Source: CAD feature listing. Evaluate the final solid. Frame: model axes, mm. Give positions to 0.01 mm unless a question says otherwise; leave off trailing zeros. Write each loop counter-clockwise with the first axis right and the second up, starting at its lowest first coordinate (ties: lowest second). Pieces come first, ordered by that corner, then holes. Notation, with made-up numbers: (-14.75, 3.5) -> (38.25, 3.5) arc R11 ccw to (38.25, 9.5) -> close; hole circle Ø8 at (41.5, -17.75). An arc over 180 degrees is marked (long way). Use a Markdown table: item, result. Add a question column.
Autodesk Inventor part; units mm, degrees
ref_plane "YZ Plane" through (0, 0, 0) normal (1, 0, 0) x (0, 1, 0)
ref_plane "XZ Plane" through (0, 0, 0) normal (0, 1, 0) x (-1, 0, 0)
ref_plane "XY Plane" through (0, 0, 0) normal (0, 0, 1) x (1, 0, 0)
sketch "Sketch1" plane through (0, 0, 0) normal (0, 1, 0) x (-1, 0, 0)
  line L0 (-10.0391, 0) -> (-100.3906, 0)
  line L1 (-110.4297, -10.0391) -> (-110.4297, -100.3906)
  line L2 (-100.3906, -110.4297) -> (-10.0391, -110.4297)
  line L3 (0, -100.3906) -> (0, -10.0391)
  arc A0 (-10.0391, -110.4297) -> (0, -100.3906) centre (-10.0391, -100.3906) ccw
  arc A1 (-110.4297, -100.3906) -> (-100.3906, -110.4297) centre (-100.3906, -100.3906) ccw
  arc A2 (-100.3906, 0) -> (-110.4297, -10.0391) centre (-100.3906, -10.0391) ccw
  arc A3 (0, -10.0391) -> (-10.0391, 0) centre (-10.0391, -10.0391) ccw
  line L4 (-23.0414, -4.0156) -> (-87.3883, -4.0156)
  line L5 (-106.4141, -23.0414) -> (-106.4141, -87.3883)
  line L6 (-87.3883, -106.4141) -> (-23.0414, -106.4141)
  line L7 (-4.0156, -87.3883) -> (-4.0156, -23.0414)
  circle A4 centre (-7.3285, -7.3285) radius 2.0078
  circle A5 centre (-7.3285, -103.1012) radius 2.0078
  circle A6 centre (-103.1012, -103.1012) radius 2.0078
  circle A7 centre (-103.1012, -7.3285) radius 2.0078
  line L8 (-6.3588, -17.3846) -> (-17.3846, -6.3588)
  line L9 (-93.0451, -6.3588) -> (-104.0709, -17.3846)
  line L10 (-104.0709, -93.0451) -> (-93.0451, -104.0709)
  line L11 (-17.3846, -104.0709) -> (-6.3588, -93.0451)
  arc A8 (-17.3846, -6.3588) -> (-23.0414, -4.0156) centre (-23.0414, -12.0156) ccw
  arc A9 (-4.0156, -23.0414) -> (-6.3588, -17.3846) centre (-12.0156, -23.0414) ccw
  arc A10 (-6.3588, -93.0451) -> (-4.0156, -87.3883) centre (-12.0156, -87.3883) ccw
  arc A11 (-23.0414, -106.4141) -> (-17.3846, -104.0709) centre (-23.0414, -98.4141) ccw
  arc A12 (-93.0451, -104.0709) -> (-87.3883, -106.4141) centre (-87.3883, -98.4141) ccw
  arc A13 (-106.4141, -87.3883) -> (-104.0709, -93.0451) centre (-98.4141, -87.3883) ccw
  arc A14 (-104.0709, -17.3846) -> (-106.4141, -23.0414) centre (-98.4141, -23.0414) ccw
  arc A15 (-87.3883, -4.0156) -> (-93.0451, -6.3588) centre (-87.3883, -12.0156) ccw
  point P0 (0, 0)
  point P1 (-4.0156, -4.0156)
  point P2 (-106.4141, -106.4141)
  point P3 (-106.4141, -4.0156)
  point P4 (-4.0156, -106.4141)
  point P5 (-4.0156, -19.7277)
  point P6 (-19.7277, -4.0156)
  point P7 (-55.2148, -55.2148)
  point P8 (-90.702, -4.0156)
  point P9 (-106.4141, -19.7277)
  point P10 (-106.4141, -90.702)
  point P11 (-90.702, -106.4141)
  point P12 (-19.7277, -106.4141)
  point P13 (-4.0156, -90.702)
  dimension "d25" = 360
extrude "Extrusion1" add sketch "Sketch1" along normal blind 3.2
properties part number "Spacer"
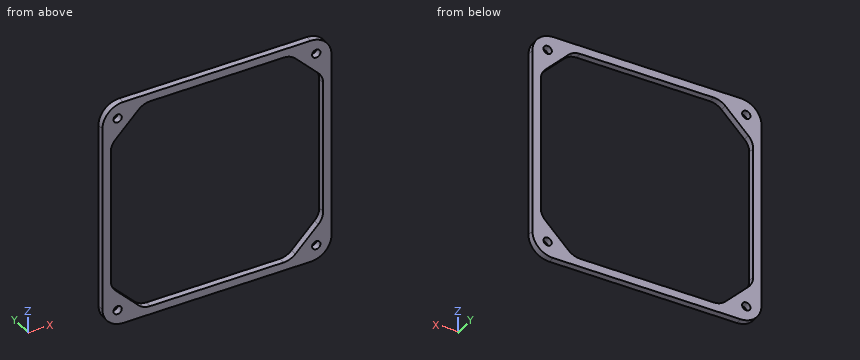
(1) Cut plane A-A on x = 66. Return the cut outline in (y, z).
(2) Material intervals for L1, parallel to X at y = 1.8, z = -79.5; L2, parallel to Z at x = 50, y = 2.75; L3, parallel to X at y = 0.2, z = -102.5, sorted ascending.
(3) Cut plane B-B on z = -28. Return the cut outline in (x, y), then the cut area to 3 significant figures.
(4) Cut plane C-C on y = 1.3. Return the cut outline in (x, z), then the cut area to 3 significant figures.
Output:
| question | item | result |
|---|---|---|
| 1 | outline | (0, -110.43) -> (3.2, -110.43) -> (3.2, -106.41) -> (0, -106.41) -> close; (0, -4.02) -> (3.2, -4.02) -> (3.2, 0) -> (0, 0) -> close |
| 2 | L1 | 0 to 4.02, 106.41 to 110.43 |
| 2 | L2 | -110.43 to -106.41, -4.02 to 0 |
| 2 | L3 | 0.22 to 5.41, 9.24 to 15.81, 94.62 to 101.19, 105.02 to 110.21 |
| 3 | outline | (0, 0) -> (4.02, 0) -> (4.02, 3.2) -> (0, 3.2) -> close; (106.41, 0) -> (110.43, 0) -> (110.43, 3.2) -> (106.41, 3.2) -> close |
| 3 | area | 25.7 mm^2 |
| 4 | outline | (0, -100.39) arc R10.04 ccw to (10.04, -110.43) -> (100.39, -110.43) arc R10.04 ccw to (110.43, -100.39) -> (110.43, -10.04) arc R10.04 ccw to (100.39, 0) -> (10.04, 0) arc R10.04 ccw to (0, -10.04) -> close; hole (4.02, -87.39) arc R8 ccw to (6.36, -93.05) -> (17.38, -104.07) arc R8 ccw to (23.04, -106.41) -> (87.39, -106.41) arc R8 ccw to (93.05, -104.07) -> (104.07, -93.05) arc R8 ccw to (106.41, -87.39) -> (106.41, -23.04) arc R8 ccw to (104.07, -17.38) -> (93.05, -6.36) arc R8 ccw to (87.39, -4.02) -> (23.04, -4.02) arc R8 ccw to (17.38, -6.36) -> (6.36, -17.38) arc R8 ccw to (4.02, -23.04) -> close; hole circle Ø4.02 at (7.33, -103.1); hole circle Ø4.02 at (7.33, -7.33); hole circle Ø4.02 at (103.1, -103.1); hole circle Ø4.02 at (103.1, -7.33) |
| 4 | area | 2,080 mm^2 |
